```python
from build123d import *

# Parameters (mm, degrees)
ESQUISSE1_W             = 149
ESQUISSE1_H             = 165
ESQUISSE1_W_2           = 100
ESQUISSE1_H_2           = 55
BOSS_EXTRU_1_DEPTH      = 1.5
CONG_1_R                = 5
ESQUISSE2_R             = 1.5
ENL_V_MAT_EXTRU_1_DEPTH = 182.045574373
ESQUISSE3_R             = 1.5
ESQUISSE3_W             = 149
ESQUISSE3_H             = 10
ESQUISSE3_H_2           = 60
ENL_V_MAT_EXTRU_2_DEPTH = 182.045574373


with BuildPart() as part:
    # Esquisse1 → Boss.-Extru.1 (new body)
    with BuildSketch(Plane.XY):
        with Locations((0, 82.5)):
            Rectangle(ESQUISSE1_W, ESQUISSE1_H)
        with Locations((0, 107.5)):
            Rectangle(ESQUISSE1_W_2, ESQUISSE1_H_2, mode=Mode.SUBTRACT)
    extrude(amount=BOSS_EXTRU_1_DEPTH)

    # Congé1
    cong_1_edges = [part.edges().sort_by_distance(p)[0] for p in [
        (-50, 135, 0.75),
        (-50, 80, 0.75),
        (50, 80, 0.75),
        (50, 135, 0.75),
    ]]
    fillet(cong_1_edges, radius=CONG_1_R)

    # Esquisse2 → Enlèv. mat.-Extru.1 (cut, through all)
    with BuildSketch(Plane.XY.offset(1.5)):
        with Locations((-30, 147.5)):
            Circle(ESQUISSE2_R)
        with Locations(Location((-30, 67.5, 0), (0, 0, 180))):
            Circle(ESQUISSE2_R)
        with Locations((30, 67.5)):
            Circle(ESQUISSE2_R)
        with Locations(Location((30, 147.5, 0), (0, 0, 180))):
            Circle(ESQUISSE2_R)
        with Locations((-55, 160)):
            Circle(ESQUISSE2_R)
        with Locations(Location((-55, 5, 0), (0, 0, 180))):
            Circle(ESQUISSE2_R)
        with Locations((55, 5)):
            Circle(ESQUISSE2_R)
        with Locations(Location((55, 160, 0), (0, 0, 180))):
            Circle(ESQUISSE2_R)
    extrude(amount=-ENL_V_MAT_EXTRU_1_DEPTH, mode=Mode.SUBTRACT)

    # Esquisse3 → Enlèv. mat.-Extru.2 (cut, through all)
    with BuildSketch(Plane.XY.offset(1.5)):
        with Locations((-68.5, 107.5)):
            Circle(ESQUISSE3_R)
        with Locations(Location((68.5, 107.5, 0), (0, 0, 180))):
            Circle(ESQUISSE3_R)
        with Locations((0, 160)):
            Rectangle(ESQUISSE3_W, ESQUISSE3_H)
        with Locations((0, 30)):
            Rectangle(ESQUISSE3_W, ESQUISSE3_H_2)
    extrude(amount=-ENL_V_MAT_EXTRU_2_DEPTH, mode=Mode.SUBTRACT)


solid = part.part
```
Geometry check sheet. Reference: the model listing, model coordinates, mm. A direction names the side the tool comes from. Coordinates: 2 decimals unless noted, no trailing zeros. Order: outer loops, then holes, each group sorted by start corner. A loop starts at its lowest first (then second) coordinate and runs counter-clockwise, first axis right, second up. Notation, with made-up numbers: M 62.5,-39 L 95.5,-39 A23 ccw 95.5,-21 Z; hole C -29,-15.5 d10. An arc over 180 degrees is marked long. One line per question, with ' | ' between items. Start each with the question number.
Item 1: Cross-section at D-D on z = 1.05. Enter the section's corners in (x, y), then the cut area to 3 significant figures.
Item 2: Material ranges on L1, parallel to Y at x = 30, z = 1.1; L2, parallel to X at y = 67.5, z = 0.75; L3, parallel to X at y = 107.5, z = 1, recorded low to high. Write a range as [from, to].
Item 3: Cross-section at C-C on y = 89. Enter the section's corners in (x, z), then the cut area to 3 significant figures.
Item 4: Draft check along X on faces 3 (the cylindrical face through (49, 133, 1)), 4 (the flat face through (-1, 140, 1.5)). Enter one of: pulls with the +X half, pulls with the -X half, needs draft (parallel to the pull), parting line crosses it, or undercut.
Item 5: Gauge pin test, flat end, axial feed: pin 1 (5 mm diameter, centred on x = -30, y = 67.5, fed in from +Z). Record the tip position at first contact, or that the pin passes through.
Item 6: Cross-section at A-A on x = -23. Enter the section's corners in (y, z).
Item 7: Cross-section at B-B on y = 147.5. Enter the section's corners in (x, z).
Item 8: Set-up check for faces 1 (the cylindrical face through (-48, 81, 1)), 2 (the flat face through (-1, 140, 0)): record each of +Z, -Z, +X, -X, +Y, -Y from which the full face is reachable in a straight line by a thin tool's end or side.
Findings:
1) outline: M -74.5,60 L 74.5,60 L 74.5,155 L -74.5,155 Z; hole C -68.5,107.5 d3; hole M -50,85 A5 ccw -45,80 L 45,80 A5 ccw 50,85 L 50,130 A5 ccw 45,135 L -45,135 A5 ccw -50,130 Z; hole C -30,67.5 d3; hole C -30,147.5 d3; hole C 30,67.5 d3; hole C 30,147.5 d3; hole C 68.5,107.5 d3 | area: 8,630 mm²
2) L1: y = [60, 66], [69, 80], [135, 146], [149, 155] | L2: x = [-74.5, -31.5], [-28.5, 28.5], [31.5, 74.5] | L3: x = [-74.5, -70], [-67, -50], [50, 67], [70, 74.5]
3) outline: M -74.5,0 L -50,0 L -50,1.5 L -74.5,1.5 Z; M 50,0 L 74.5,0 L 74.5,1.5 L 50,1.5 Z | area: 73.5 mm²
4) face 3: undercut | face 4: needs draft
5) pin 1: stops at z = 1.5
6) outline: M 60,0 L 80,0 L 80,1.5 L 60,1.5 Z; M 135,0 L 155,0 L 155,1.5 L 135,1.5 Z
7) outline: M -74.5,0 L -31.5,0 L -31.5,1.5 L -74.5,1.5 Z; M -28.5,0 L 28.5,0 L 28.5,1.5 L -28.5,1.5 Z; M 31.5,0 L 74.5,0 L 74.5,1.5 L 31.5,1.5 Z
8) face 1: +Z, -Z | face 2: -Z, +X, -X, +Y, -Y
